Source: CAD feature listing. Evaluate the final solid. Frame: model axes, mm. Give positions to 0.01 mm unless a question says otherwise; leave off trailing zeros. Order: outer loops, then holes, each group sorted by start corner. A loop starts at its lowest first (then second) coordinate and runs counter-clockwise, first axis right, second up. Notation, with made-up numbers: M -19.5,23.5 L 31.5,23.5 A17 ccw 31.5,49.5 Z; hole C 14.25,-8 d8. An arc over 180 degrees is marked long. Answer as a JSON object with one key per item and string values. Group by question number.
1. Section query C-C (x = -26.5). Output: boundary loops of the cut face in (y, z).
2. Material intervals for L1, parallel to X at y = -18, z = 25; L2, parallel to X at y = -15.5, z = 48; L3, parallel to Z at x = -52, y = -11.5, sorted ascending. Write a range as [from, to].
3. Pin query (flat end, axial travel): P1, Ø12, axis at y = -13, z = 18.5, coming from the +X side; P2, Ø3, axis at x = -25, z = 8, coming from the +Y side; P3, Ø6, axis at x = -76.5, y = -19, coming from the +Z side; P4, Ø1, axis at x = -28, y = -6.5, coming from the +Z side. Return the tip coordinate at first contact, or that it passes through.
4. Section query A-A (y = -15.5). Output: boundary loops of the cut face in (x, z).
5. Section query B-B (z = 14.5). Output: boundary loops of the cut face in (x, y).
from build123d import *

# Parameters (mm, degrees)
F1_DEPTH = 25


with BuildPart() as f1:
    # F0 (on Front) → F1 (new body)
    with BuildSketch(Plane.XZ):
        with BuildLine():
            ThreePointArc((-12.9923656989, 28.902602186), (-12.9909523706, 29.0967337225), (-12.9904812574, 29.290869832))
            ThreePointArc((-12.9904812574, 29.290869832), (-12.9945641617, 29.8623728238), (-13.0068120409, 30.4337591459))
            Line((-13.0068120409, 30.4337591459), (-32.6551738333, 63.7361201862))
            ThreePointArc((-32.6551738333, 63.7361201862), (-33.3181920134, 64.1190342382), (-33.9884178287, 64.489187767))
            Line((-33.9884178287, 64.489187767), (-72.6532893918, 64.1243878322))
            ThreePointArc((-72.6532893918, 64.1243878322), (-73.3164117783, 63.741654271), (-73.9720870452, 63.3462984531))
            Line((-73.9720870452, 63.3462984531), (-92.988596816, 29.679137478))
            ThreePointArc((-92.988596816, 29.679137478), (-92.9887010223, 28.9134898649), (-92.974150474, 28.1479805181))
            Line((-92.974150474, 28.1479805181), (-73.3257886816, -5.1543805222))
            ThreePointArc((-73.3257886816, -5.1543805222), (-72.6627705014, -5.5372945741), (-71.9925446861, -5.9074481029))
            Line((-71.9925446861, -5.9074481029), (-33.3276731231, -5.5426481682))
            ThreePointArc((-33.3276731231, -5.5426481682), (-32.6645507366, -5.1599146069), (-32.0088754696, -4.764558789))
            Line((-32.0088754696, -4.764558789), (-12.9923656989, 28.902602186))
        make_face()
        with BuildLine():
            ThreePointArc((-13.0068120409, 30.4337591459), (-12.9945641617, 29.8623728238), (-12.9904812574, 29.290869832))
            ThreePointArc((-12.9904812574, 29.290869832), (-12.9909523706, 29.0967337225), (-12.9923656989, 28.902602186))
            Line((-12.9923656989, 28.902602186), (-12.5575819284, 29.6723509657))
            Line((-12.5575819284, 29.6723509657), (-13.0068120409, 30.4337591459))
        make_face()
        with BuildLine():
            ThreePointArc((-33.9884178287, 64.489187767), (-33.3181920134, 64.1190342382), (-32.6551738333, 63.7361201862))
            Line((-32.6551738333, 63.7361201862), (-33.1044039458, 64.4975283665))
            Line((-33.1044039458, 64.4975283665), (-33.9884178287, 64.489187767))
        make_face()
        with BuildLine():
            Line((-32.4436592401, -5.5343075687), (-32.0088754696, -4.764558789))
            ThreePointArc((-32.0088754696, -4.764558789), (-32.6645507366, -5.1599146069), (-33.3276731231, -5.5426481682))
            Line((-33.3276731231, -5.5426481682), (-32.4436592401, -5.5343075687))
        make_face()
        with BuildLine():
            ThreePointArc((-73.9720870452, 63.3462984531), (-73.3164117783, 63.741654271), (-72.6532893918, 64.1243878322))
            Line((-72.6532893918, 64.1243878322), (-73.5373032748, 64.1160472328))
            Line((-73.5373032748, 64.1160472328), (-73.9720870452, 63.3462984531))
        make_face()
        with BuildLine():
            Line((-72.8765585691, -5.9157887024), (-71.9925446861, -5.9074481029))
            ThreePointArc((-71.9925446861, -5.9074481029), (-72.6627705014, -5.5372945741), (-73.3257886816, -5.1543805222))
            Line((-73.3257886816, -5.1543805222), (-72.8765585691, -5.9157887024))
        make_face()
        with BuildLine():
            ThreePointArc((-92.974150474, 28.1479805181), (-92.9887010223, 28.9134898649), (-92.988596816, 29.679137478))
            Line((-92.988596816, 29.679137478), (-93.4233805865, 28.9093886984))
            Line((-93.4233805865, 28.9093886984), (-92.974150474, 28.1479805181))
        make_face()
    extrude(amount=F1_DEPTH)


solid = f1.part
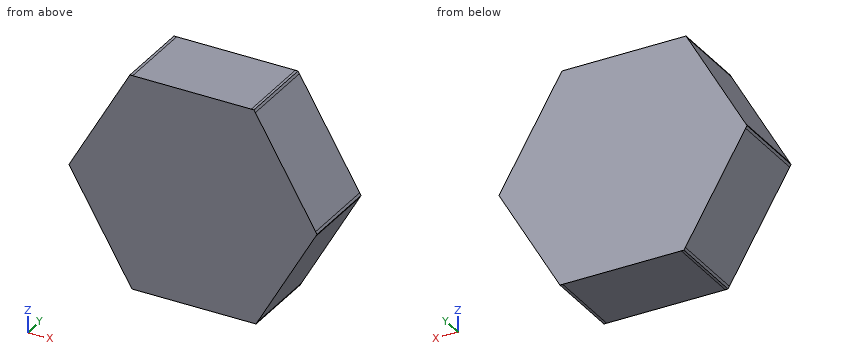
Answer sheet:
{
 "1": {"outline": "M -25,4.99 L 0,4.99 L 0,53.3 L -25,53.3 Z"},
 "2": {"L1": "[-91.12, -15.2]", "L2": "[-82.64, -23.37]", "L3": "[-5.72, 64.32]"},
 "3": {"P1": "x = -15.48", "P2": "y = 0", "P3": "z = 64.12", "P4": "z = 56.69"},
 "4": {"outline": "M -93.42,28.91 L -72.88,-5.92 L -32.44,-5.53 L -12.56,29.67 L -33.1,64.5 L -73.54,64.12 Z"},
 "5": {"outline": "M -84.92,-25 L -21.13,-25 L -21.13,0 L -84.92,0 Z"}
}
